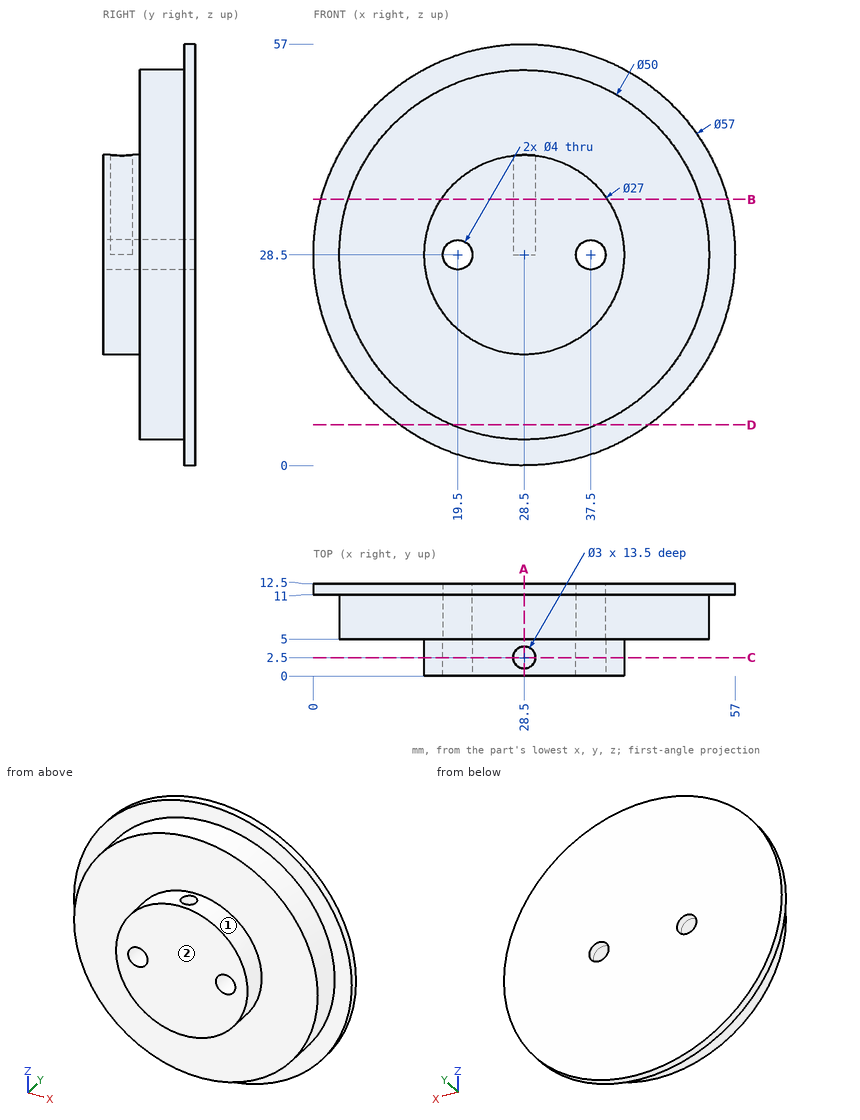
Here's the drawing with two shaded views (mm, measured from the low corner). I have some questions. A direction names the side the tool comes from. Round coordinates to 2 decimals unless told otherwise and drop trailing zeros. Loops run counter-clockwise (first coordinate to the right, second up) from the corner with the lowest first, then second, coordinate; pieces in that order, holes last.
Item 1: Please list where these lines run through material, in increasing order: L1, parallel to X at y = 12.2, z = 28.5; L2, parallel to X at y = 6.75, z = 28.5; L3, parallel to Y at x = 8.5, z = 23.5.
Item 2: Suppose I cut it at D-D, the plane z = 5.5. Write out the boundary of the cut face in (x, y).
Item 3: Which directions (+Z, -Z, +X, -X, +Y, -Y) give clear straight access to the entire face, cutting with the end or side of a thin tool? Please do the marked faces 1 and 2.
Item 4: Suppose I cut it at A-A, the plane x = 28.5. Write out the boundary of the cut face in (y, z), then the cut area to 3 significant figures.
Item 5: Will these pins go through, and if not, where does the flat tip stop? pin 1 Ø1 at (y, z) = (6.5, 39.5) entering from +X; pin 2 Ø5 at (y, z) = (4, 21) entering from +X; pin 3 Ø3.5 at (x, y) = (28.5, 2.5) entering from +Z; pin 4 Ø3 at (x, z) = (19.5, 28.5) entering from -Y.
Item 6: Suppose I cut it at C-C, the plane y = 2.5. Write out the boundary of the cut face in (x, z), then the cut area to 3 significant figures.
Item 7: Suppose I cut it at B-B, the plane z = 36. Write out the boundary of the cut face in (x, y), then the cut area to 3 significant figures.
Reported:
1. L1: x = 0 to 17.5, 21.5 to 35.5, 39.5 to 57
1. L2: x = 3.5 to 17.5, 21.5 to 35.5, 39.5 to 53.5
1. L3: y = 5 to 12.5
2. outline: (11.67, 11) - (18.7, 11) - (18.7, 5) - (38.3, 5) - (38.3, 11) - (45.33, 11) - (45.33, 12.5) - (11.67, 12.5) - close
3. face 1: -Y
3. face 2: +Z, -Z, +X, -X, -Y
4. outline: (0, 15) - (5, 15) - (5, 3.5) - (11, 3.5) - (11, 0) - (12.5, 0) - (12.5, 57) - (11, 57) - (11, 53.5) - (5, 53.5) - (5, 42) - (4, 42) - (4, 28.5) - (1, 28.5) - (1, 42) - (0, 42) - close
4. area: 480 mm2
5. pin 1: stops at x = 51.19
5. pin 2: stops at x = 52.95
5. pin 3: stops at z = 42
5. pin 4: passes through
6. outline: (27, 28.5) - (27, 41.92) arc R13.5 ccw (long way) to (30, 41.92) - (30, 28.5) - close; hole circle Ø4 at (19.5, 28.5); hole circle Ø4 at (37.5, 28.5)
6. area: 507 mm2
7. outline: (1, 11) - (4.65, 11) - (4.65, 5) - (17.28, 5) - (17.28, 0) - (39.72, 0) - (39.72, 5) - (52.35, 5) - (52.35, 11) - (56, 11) - (56, 12.5) - (1, 12.5) - close; hole circle Ø3 at (28.5, 2.5)
7. area: 474 mm2
